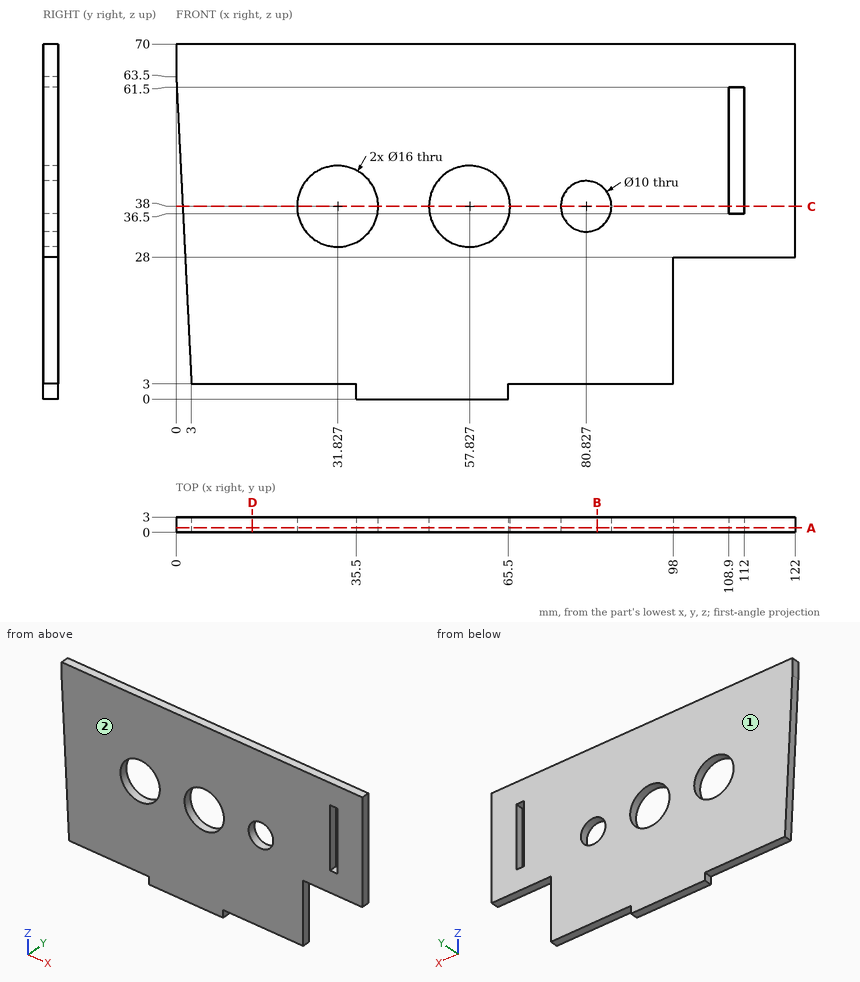
Part print with two shaded views. Sizes in mm from the minimum x, y, z corner. Coordinates: 2 decimals unless noted, no trailing zeros. Write each loop counter-clockwise with the first axis right and the second up, starting at its lowest first coordinate (ties: lowest second). Pieces come first, ordered by that corner, then holes.
(1) Mould opens along Y. For the marked faces 1 and 2 say: pulls with the +Y half, pulls with the -Y half, needs draft (parallel to the pull), parting line crosses it, or undercut.
(2) Cut at A-A on y = 0.85. List the corners of the cut face in (x, z), and give its area (3 significant figures).
(3) Cut at C-C on z = 38. List the corners of the cut face in (x, y), and give its area (3 significant figures).
(4) Cut at B-B on x = 83. List the corners of the cut face in (y, z).
(5) Cut at D-D on x = 15. List the corners of the cut face in (y, z), and give its area (3 significant figures).
(6) Pin check, flat tips, straight feed: pin 1 Ø1.5 at (y, z) = (1, 1.5) entering from -X; pin 2 Ø0.9 at (x, y) = (76.5, 2) entering from -Z; pin 3 Ø1.5 at (y, z) = (1, 1.5) entering from +X; pin 4 Ø13 at (x, z) = (57.83, 38) entering from -Y. Stop position of each tip, or through.
(7) Drill centre lines: line 1 (X direction, y = 1.2, z = 40.5); line 2 (Z direction, x = 66, y = 0.65); line 3 (Z direction, x = 64.5, y = 0.7). Where is each one in solid material? Low to high.
Working result:
1. face 1: pulls with the +Y half
1. face 2: pulls with the -Y half
2. outline: (0, 63.5) - (3, 3) - (35.5, 3) - (35.5, 0) - (65.5, 0) - (65.5, 3) - (98, 3) - (98, 28) - (122, 28) - (122, 70) - (0, 70) - close; hole circle Ø16 at (31.83, 38); hole circle Ø16 at (57.83, 38); hole circle Ø10 at (80.83, 38); hole (108.9, 36.5) - (112, 36.5) - (112, 61.5) - (108.9, 61.5) - close
2. area: 7,020 mm2
3. outline: (1.26, 0) - (23.83, 0) - (23.83, 3) - (1.26, 3) - close; (39.83, 0) - (49.83, 0) - (49.83, 3) - (39.83, 3) - close; (65.83, 0) - (75.83, 0) - (75.83, 3) - (65.83, 3) - close; (85.83, 0) - (108.9, 0) - (108.9, 3) - (85.83, 3) - close; (112, 0) - (122, 0) - (122, 3) - (112, 3) - close
3. area: 227 mm2
4. outline: (0, 3) - (3, 3) - (3, 33.5) - (0, 33.5) - close; (0, 42.5) - (3, 42.5) - (3, 70) - (0, 70) - close
5. outline: (0, 3) - (3, 3) - (3, 70) - (0, 70) - close
5. area: 201 mm2
6. pin 1: stops at x = 35.5
6. pin 2: stops at z = 3
6. pin 3: stops at x = 65.5
6. pin 4: passes through
7. line 1: x = 1.14 to 24.23, 39.43 to 50.23, 65.43 to 76.5, 85.16 to 108.9, 112 to 122
7. line 2: z = 3 to 70
7. line 3: z = 0 to 33.59, 42.41 to 70
